Source: CAD feature listing. Evaluate the final solid. Frame: model axes, mm. Face numbers are marked on the shaded views. A direction names the side the tool comes from. Coordinates: 2 decimals unless noted, no trailing zeros. Loops run counter-clockwise (first coordinate to the right, second up) from the corner with the lowest first, then second, coordinate; pieces in that order, holes last. Notation, with made-up numbers: M -16.75,-21 L 31.25,-21 A14 cw 31.25,-9 Z; hole C 51.25,1.25 d9. An arc over 180 degrees is marked long. One line per question, with ' | ' between items. Start each with the question number.
1. Access query for the marked faces 4, 5 and 6. Directions: +Z, -Z, +X, -X, +Y, -Y. A direction counts if a zero-diameter tool reaches every point of the face in a straight line with its end or side. Return the directions, or none.
2. Section query D-D, the plane z = 43. Output: boundary loops of the cut face in (x, y).
3. Section query A-A, the plane z = -62. Output: boundary loops of the cut face in (x, y), and give its area (3 significant figures).
4. Section query C-C, the plane y = -3. Output: boundary loops of the cut face in (x, z).
5. Mould query, pull axis Y, two halves, no side actions, for the marked faces 1, 2 and 3. Classes: pulls with the +Y half, pulls with the -Y half, needs draft (parallel to the pull), parting line crosses it, or undercut.
6. Section query B-B, the plane x = 2.5. Output: boundary loops of the cut face in (y, z), and give its area (3 significant figures).
7. Pin query (flat end, axial travel): P1, Ø4, axis at x = 5, y = -16, coming from the -Z side; P2, Ø10.5, axis at x = 2, z = -65.5, coming from the -Y side; P3, Ø8, axis at x = -15, y = -9.5, coming from the +Z side; P4, Ø5, axis at x = 21.5, y = 0, coming from the +Z side. Return the tip coordinate at first contact, or that it passes through.
8. Ray query, probe 1 along Y at (x, z) = (-24, 31); probe 2 along Z at (x, y) = (0, 2); probe 3 along Z at (x, y) = (0, 16.5). Return the intervals inside material, ascending.
```python
from build123d import *

# Parameters (mm, degrees)
SKETCH001_W  = 20
SKETCH001_H  = 80.939507
PAD001_DEPTH = 40
SKETCH_R     = 12.5
PAD_DEPTH    = 20
SKETCH002_R  = 10
PAD002_DEPTH = 6
SKETCH003_R  = 17.5
POCKET_DEPTH = 6


with BuildPart() as pad001:
    # Sketch001 → Pad001 (new body, symmetric)
    with BuildSketch(Plane.YZ):
        with Locations((0, 50.469753)):
            Rectangle(SKETCH001_W, SKETCH001_H)
    extrude(amount=PAD001_DEPTH, both=True)


with BuildPart() as cut:
    # Sketch → Pad (new body, symmetric)
    with BuildSketch(Plane.XZ):
        with BuildLine():
            Line((30, 40), (30, 0))
            Line((30, 0), (-30, 0))
            Line((-30, 0), (-30, 40))
            ThreePointArc((30, 40), (0, 70), (-30, 40))
        make_face()
        with Locations((0, 40)):
            Circle(SKETCH_R, mode=Mode.SUBTRACT)
    extrude(amount=PAD_DEPTH, both=True)

    # Cut: cut Pad001
    add(pad001.part, mode=Mode.SUBTRACT)


with BuildPart() as fusion:
    # Sketch002 → Pad002 (new body, symmetric)
    with BuildSketch(Plane.XZ):
        Polygon((-30, 0), (-30, -75), (-18, -87), (18, -87), (30, -75), (30, 0), align=None)
        with Locations((0, -62)):
            Circle(SKETCH002_R, mode=Mode.SUBTRACT)
    extrude(amount=PAD002_DEPTH, both=True)

    # Sketch003 → Pocket (cut)
    with BuildSketch(Plane.XZ.offset(6)):
        with Locations((0, -62)):
            Circle(SKETCH003_R)
    extrude(amount=-POCKET_DEPTH, mode=Mode.SUBTRACT)

    # Fusion: union Cut
    add(cut.part)


solid = fusion.part
```
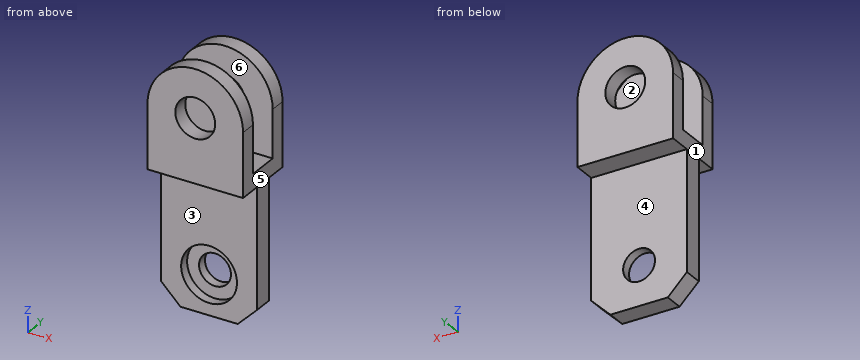
Taken from the geometry:
1) face 4: -Z, +X, -X, +Y | face 5: +Z, -Z, +X, +Y, -Y | face 6: +Z, +X, -X
2) outline: M -29.85,-20 L -12.13,-20 L -12.13,-10 L -29.85,-10 Z; M -29.85,10 L -12.13,10 L -12.13,20 L -29.85,20 Z; M 12.13,-20 L 29.85,-20 L 29.85,-10 L 12.13,-10 Z; M 12.13,10 L 29.85,10 L 29.85,20 L 12.13,20 Z
3) outline: M -30,-6 L -17.5,-6 L -17.5,0 L -10,0 L -10,6 L -30,6 Z; M 10,0 L 17.5,0 L 17.5,-6 L 30,-6 L 30,6 L 10,6 Z | area: 390 mm^2
4) outline: M -30,-75 L -18,-87 L 18,-87 L 30,-75 L 30,10 L -30,10 Z; hole C 0,-62 d35
5) face 1: needs draft | face 2: undercut | face 3: pulls with the -Y half
6) outline: M -20,0 L -6,0 L -6,-44.68 L 0,-44.68 L 0,-52.32 L 6,-52.32 L 6,0 L 20,0 L 20,27.75 L 10,27.75 L 10,10 L -10,10 L -10,27.75 L -20,27.75 Z; M -20,52.25 L -10,52.25 L -10,69.9 L -20,69.9 Z; M -6,-87 L 6,-87 L 6,-71.68 L 0,-71.68 L 0,-79.32 L -6,-79.32 Z; M 10,52.25 L 20,52.25 L 20,69.9 L 10,69.9 Z | area: 1,830 mm^2
7) P1: z = 0 | P2: through | P3: z = 67.9 | P4: z = 10
8) probe 1: -20 to -10, 10 to 20 | probe 2: -87 to -72, -52 to 10 | probe 3: 0 to 27.5, 52.5 to 70
